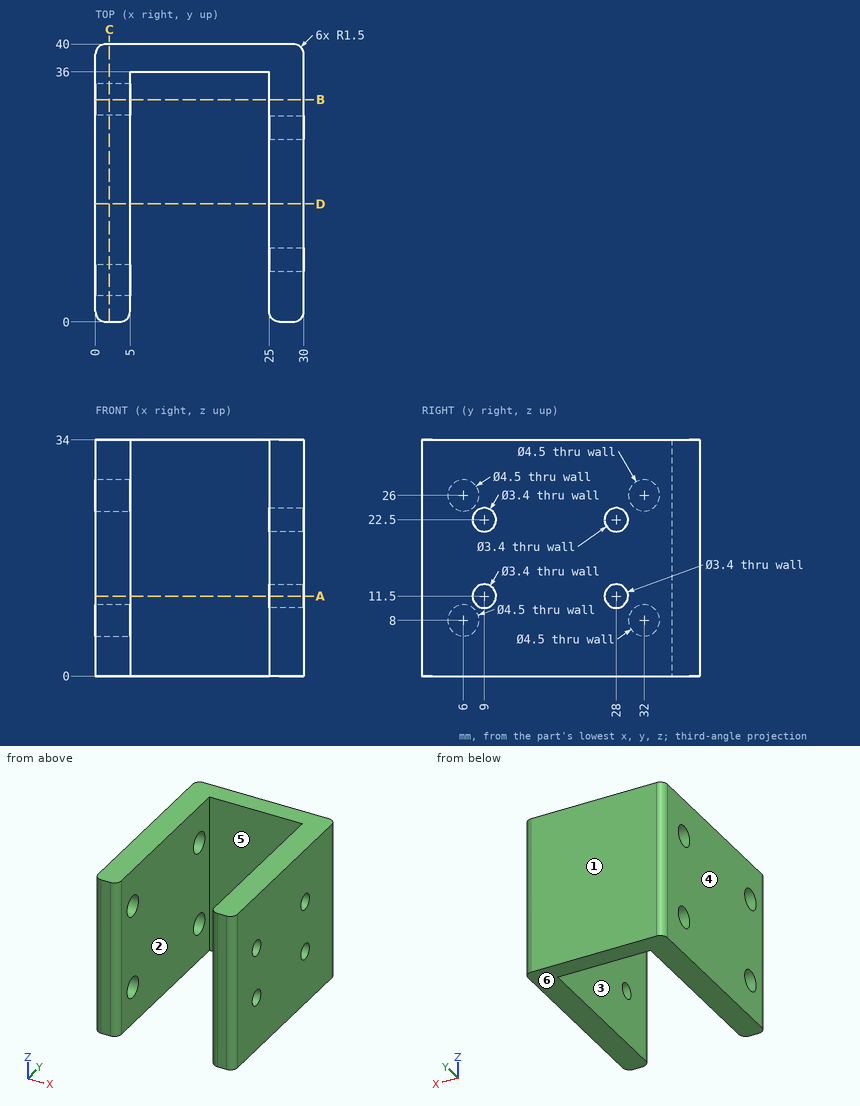
Answer from the drawing. Dimensions are ordinates in mm from the lowest x, y and z of the part. A direction names the side the tool comes from. Coordinates: 2 decimals unless noted, no trailing zeros. Loops run counter-clockwise (first coordinate to the right, second up) from the corner with the lowest first, then second, coordinate; pieces in that order, holes last.
Q1. Each of these flat-tipped pins is pushed along its axis until it touches: pin 1 Ø6 at (y, z) = (32, 26) entering from -X; pin 2 Ø6 at (x, z) = (12, 30.5) entering from -Y; pin 3 Ø3 at (y, z) = (9, 22.5) entering from +X. Where does it stop, or does it pass through?
Q2. The part is cut by section C-C on x = 2. Write down the section's boundary in (y, z), and give its area (3 significant figures).
Q3. The part is cut by section B-B on y = 32. Write down the section's boundary in (x, z), and give its area (3 significant figures).
Q4. The mould has two halves that part along X. Classify the marked faces 3, 4, 5 and 6: +X half, -X half, draft (parallel to the pull), parting line (faces both ways), or undercut.
Q5. The part is cut by section A-A on z = 11.5. Write down the section's boundary in (x, y).
Q6. Consider probe 1 along Y at (x, z) = (27.45, 11.5); probe 2 along X at (y, z) = (9, 8.5); probe 3 along Y at (x, z) = (1.8, 26). Determine where each line is inside the solid, lowest interval first.
Q7. The part is cut by section D-D on y = 17. Write down the section's boundary in (x, z).
Q8. Which of the six approach directions +Z, -Z, +X, -X, +Y, -Y give full straight-line access (tool end or side, diameter ignored) to the marked faces 1 and 2?
Results below:
1. pin 1: stops at x = 0
1. pin 2: stops at y = 36
1. pin 3: stops at x = 5
2. outline: (0, 0) - (40, 0) - (40, 34) - (0, 34) - close; hole circle Ø4.5 at (6, 8); hole circle Ø4.5 at (6, 26); hole circle Ø4.5 at (32, 8); hole circle Ø4.5 at (32, 26)
2. area: 1,300 mm2
3. outline: (0, 0) - (5, 0) - (5, 5.75) - (0, 5.75) - close; (0, 10.25) - (5, 10.25) - (5, 23.75) - (0, 23.75) - close; (0, 28.25) - (5, 28.25) - (5, 34) - (0, 34) - close; (25, 0) - (30, 0) - (30, 34) - (25, 34) - close
3. area: 295 mm2
4. face 3: undercut
4. face 4: -X half
4. face 5: undercut
4. face 6: draft
5. outline: (0, 1.5) arc R1.5 ccw to (1.5, 0) - (3.5, 0) arc R1.5 ccw to (5, 1.5) - (5, 36) - (25, 36) - (25, 29.7) - (30, 29.7) - (30, 38.5) arc R1.5 ccw to (28.5, 40) - (1.5, 40) arc R1.5 ccw to (0, 38.5) - close; (25, 1.5) arc R1.5 ccw to (26.5, 0) - (28.5, 0) arc R1.5 ccw to (30, 1.5) - (30, 7.3) - (25, 7.3) - close; (25, 10.7) - (30, 10.7) - (30, 26.3) - (25, 26.3) - close
6. probe 1: y = 0 to 7.3, 10.7 to 26.3, 29.7 to 40
6. probe 2: x = 0 to 5, 25 to 30
6. probe 3: y = 0 to 3.75, 8.25 to 29.75, 34.25 to 40
7. outline: (0, 0) - (5, 0) - (5, 34) - (0, 34) - close; (25, 0) - (30, 0) - (30, 34) - (25, 34) - close
8. face 1: +Z, -Z, +X, -X, +Y
8. face 2: +Z, -Z, -Y
